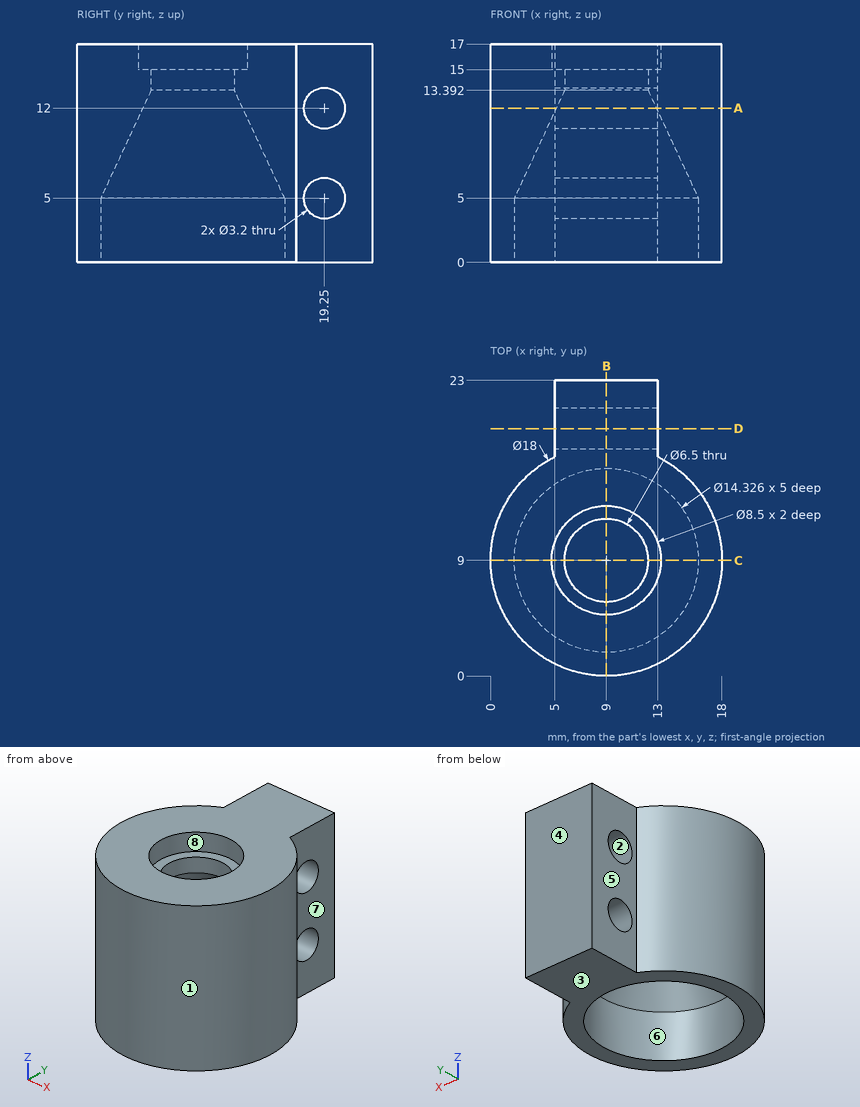
Verification items for this drawing (mm, ordinates from the low corner). A direction names the side the tool comes from. Give positions to 0.01 mm unless a question says otherwise; leave off trailing zeros. Order: outer loops, then holes, each group sorted by start corner. A loop starts at its lowest first (then second) coordinate and runs counter-clockwise, first axis right, second up.
1) Gauge pin test, flat ends, axial feed: pin 1 (5 mm diameter, centred on y = 19, z = 11.5, fed in from -X) (1 decimal); pin 2 (6 mm diameter, centred on y = 3, z = 10, fed in from -X) (1 decimal); pin 3 (6 mm diameter, centred on x = 9, y = 9, fed in from +Z); pin 4 (1.5 mm diameter, centred on x = 3.5, z = 8.5, fed in from +Y) (1 decimal). Record the tip position at first contact, or that the pin passes through.
Results are:
pin 1: stops at x = 4
pin 2: stops at x = 0.5
pin 3: passes through
pin 4: stops at y = 16.6
2) Material ranges on probe 1 along X at (y, z) = (9.25, 1.5); probe 2 along Z at (x, y) = (5.75, 20.5); probe 3 along Z at (x, y) = (9.5, 19), recorded low to high.
Results are:
probe 1: x = 0 to 1.84, 16.16 to 18
probe 2: z = 0 to 4, 6 to 11, 13 to 17
probe 3: z = 0 to 3.42, 6.58 to 10.42, 13.58 to 17
3) Cross-section at C-C (y = 9). Record the boundary of the cut face in (x, z).
Results are:
outline: (0, 0) - (1.84, 0) - (1.84, 5) - (5.75, 13.39) - (5.75, 15) - (4.75, 15) - (4.75, 17) - (0, 17) - close; (12.25, 13.39) - (16.16, 5) - (16.16, 0) - (18, 0) - (18, 17) - (13.25, 17) - (13.25, 15) - (12.25, 15) - close
4) Cross-section at D-D (y = 19.25). Record the boundary of the cut face in (x, z).
Results are:
outline: (5, 0) - (13, 0) - (13, 3.4) - (5, 3.4) - close; (5, 6.6) - (13, 6.6) - (13, 10.4) - (5, 10.4) - close; (5, 13.6) - (13, 13.6) - (13, 17) - (5, 17) - close
5) Cross-section at B-B (x = 9). Record the boundary of the cut face in (y, z).
Results are:
outline: (0, 0) - (1.84, 0) - (1.84, 5) - (5.75, 13.39) - (5.75, 15) - (4.75, 15) - (4.75, 17) - (0, 17) - close; (12.25, 13.39) - (16.16, 5) - (16.16, 0) - (23, 0) - (23, 17) - (13.25, 17) - (13.25, 15) - (12.25, 15) - close; hole circle Ø3.2 at (19.25, 5); hole circle Ø3.2 at (19.25, 12)
6) Tool access check on the marked faces 5, 6, 7 and 8. Record the directions out of +Z, -Z, +X, -X, +Y, -Y that give a thin tool (end or side, any length) a straight path to the whole face; none if there is none.
Results are:
face 5: +Z, -Z, -X, +Y
face 6: -Z
face 7: +Z, -Z, +X, +Y
face 8: +Z
7) Draft check along Y on the marked faces 1, 2, 3 and 4. Enter one of: released by +Y, released by -Y, zero draft, split by the parting line, or undercut.
Results are:
face 1: split by the parting line
face 2: undercut
face 3: zero draft
face 4: released by +Y
8) Cross-section at A-A (z = 12). Record the boundary of the cut face in (x, y).
Results are:
outline: (5, 17.06) arc R9 ccw (long way) to (13, 17.06) - (13, 17.65) - (5, 17.65) - close; (5, 20.85) - (13, 20.85) - (13, 23) - (5, 23) - close; hole circle Ø7.8 at (9, 9)
